from build123d import *

# Parameters (mm, degrees)
F0_R     = 25.4
F1_DEPTH = 40.2336
F0_R_2   = 9.525
F2_DEPTH = 15.7734


with BuildPart() as f1:
    # F0 (on Top) → F1 (new body)
    with BuildSketch(Plane.XY):
        with BuildLine():
            Line((-25.28207, 27.642332), (-26.324773, 27.894657))
            ThreePointArc((-26.324773, 27.894657), (-61.096783, -0.281283), (-25.776829, -27.767227))
            ThreePointArc((-25.776829, -27.767227), (-10.058643, -17.660062), (-3.948128, 0))
            ThreePointArc((-3.948128, 0), (-9.901856, 17.458777), (-25.28207, 27.642332))
        make_face()
        with Locations((-32.523148, 0)):
            Circle(F0_R, mode=Mode.SUBTRACT)
        with Locations((-32.523148, 0)):
            Circle(F0_R)
        with BuildLine():
            ThreePointArc((-18.843367, -4.122653), (-46.810648, 0), (-18.843367, 4.122653))
            Line((-18.843367, 4.122653), (-13.386128, 4.122653))
            Line((-13.386128, 4.122653), (-13.386128, -4.122653))
            Line((-13.386128, -4.122653), (-18.843367, -4.122653))
        make_face(mode=Mode.SUBTRACT)
    extrude(amount=F1_DEPTH)

    # F0 (on Top) → F2 (join)
    with BuildSketch(Plane.XY):
        with BuildLine():
            ThreePointArc((-3.948128, 0), (-10.058643, -17.660062), (-25.776829, -27.767227))
            Line((-25.776829, -27.767227), (24.059165, -15.659087))
            Line((24.059165, -15.659087), (26.318371, -15.110191))
            ThreePointArc((26.318371, -15.110191), (37.314952, 0.589055), (25.184714, 15.429824))
            Line((25.184714, 15.429824), (-25.28207, 27.642332))
            ThreePointArc((-25.28207, 27.642332), (-9.901856, 17.458777), (-3.948128, 0))
        make_face()
        with Locations((21.450878, 0.000175)):
            Circle(F0_R_2, mode=Mode.SUBTRACT)
    extrude(amount=F2_DEPTH)


solid = f1.part
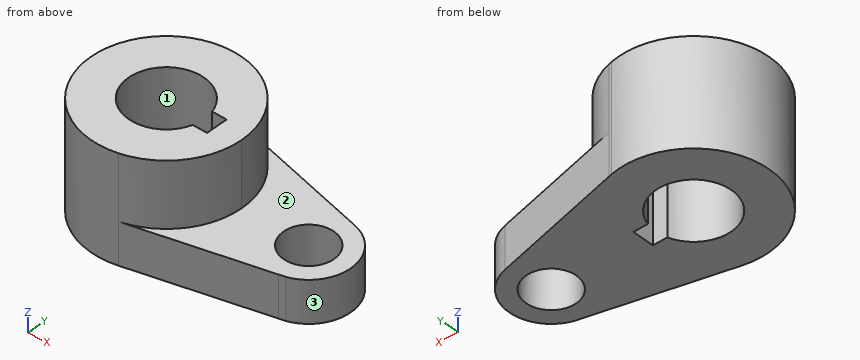
Model file for the job. Use its own axes, mm. Face numbers are marked on the shaded views. Give positions to 0.01 mm unless a question says otherwise; leave off trailing zeros. Loops run counter-clockwise (first coordinate to the right, second up) from the corner with the lowest first, then second, coordinate; pieces in that order, holes last.
Item 1: Slice it at D-D (z = 4). Give the number of separate pieces and of enclosed holes in the cut face, plus the area to 3 significant figures.
Check values:
separate pieces: 1
enclosed holes: 2
area: 3,180 mm2
Item 2: Slice it at A-A (z = 18). Write the cut outline in (x, y) (1 decimal), plus the area to 3 significant figures.
Check values:
outline: (-26.3, 27.9) arc R28.6 ccw (long way) to (-25.8, -27.8) arc R28.6 ccw to (-3.9, 0) arc R28.6 ccw to (-25.3, 27.6) - close; hole (-18.8, -4.1) - (-13.4, -4.1) - (-13.4, 4.1) - (-18.8, 4.1) arc R14.3 ccw (long way) to start
area: 1,880 mm2
Item 3: Drop flat-ended pins along their axis: P1, Ø6, axis at y = -19, z = 23, coming from the +X side; P2, Ø12, axis at x = -25, z = 7, coming from the -Y side; P3, Ø2.5, axis at x = -16.5, z = 27, coming from the +Y side; P4, Ø9, axis at y = -1, z = 21, coming from the -X side. Give the stop position or say it passes through.
Check values:
P1: stops at x = -8.85
P2: stops at y = -28.53
P3: stops at y = 24.46
P4: stops at x = -61.1
Item 4: Drill centre lines: line 1 along X through (y, z) = (-8, 9.5); line 2 along Y through (x, z) = (-31, 26); line 3 along X through (y, z) = (-3, 7.5). Where is each one in solid material? Low to high.
Check values:
line 1: x = -59.96 to -44.36, -20.69 to 16.28, 26.62 to 35.16
line 2: y = -28.53 to -14.21, 14.21 to 28.53
line 3: x = -60.94 to -46.49, -13.39 to 12.41, 30.49 to 37.04
Item 5: Slice it at C-C (y = 10.5). Write the cut outline in (x, z).
Check values:
outline: (-59.1, 0) - (-42.21, 0) - (-42.21, 40.23) - (-59.1, 40.23) - close; (-22.83, 0) - (33.36, 0) - (33.36, 15.77) - (-5.95, 15.77) - (-5.95, 40.23) - (-22.83, 40.23) - close
Item 6: Mould opens along X. For the marked faces 1, 2 and 3 say: +X half, -X half, draft (parallel to the pull), parting line (faces both ways), or undercut.
Check values:
face 1: undercut
face 2: draft
face 3: +X half
Item 7: Slice it at B-B (x = 29.5). Write the cut outline in (y, z).
Check values:
outline: (-13.68, 0) - (-5.09, 0) - (-5.09, 15.77) - (-13.68, 15.77) - close; (5.09, 0) - (13.68, 0) - (13.68, 15.77) - (5.09, 15.77) - close
